from build123d import *

# Parameters (mm, degrees)
SKETCH1_W            = 97.5
SKETCH1_H            = 35
BOSS_EXTRUDE1_DEPTH  = 22
SKETCH2_R            = 3
BOSS_EXTRUDE2_DEPTH  = 4
BOSS_EXTRUDE3_DEPTH  = 2
BOSS_EXTRUDE4_DEPTH  = 8
SKETCH6_R            = 5
BOSS_EXTRUDE5_DEPTH  = 4
SKETCH7_R            = 6.5
SKETCH7_R_2          = 3
BOSS_EXTRUDE6_DEPTH  = 1.5
BOSS_EXTRUDE8_DEPTH  = 8
BOSS_EXTRUDE9_DEPTH  = 4
SKETCH14_R           = 4
BOSS_EXTRUDE10_DEPTH = 2
SKETCH20_R           = 5
BOSS_EXTRUDE11_DEPTH = 4
SKETCH21_R           = 6
SKETCH21_R_2         = 3
BOSS_EXTRUDE12_DEPTH = 1.5
SKETCH22_R           = 2
CUT_EXTRUDE1_DEPTH   = 28.5
SKETCH25_R           = 1.5
CUT_EXTRUDE3_DEPTH   = 39


with BuildPart() as part:
    # Sketch1 → Boss-Extrude1 (new body)
    with BuildSketch(Plane.XY):
        Rectangle(SKETCH1_W, SKETCH1_H)
    extrude(amount=BOSS_EXTRUDE1_DEPTH)

    # Sketch2 → Boss-Extrude2 (add)
    with BuildSketch(Plane(origin=(0, 17.5, 0), x_dir=(1, 0, 0), z_dir=(0, 1, 0))):
        with Locations((-36.875, -11)):
            Circle(SKETCH2_R)
        with Locations((36.875, -11)):
            Circle(SKETCH2_R)
    extrude(amount=BOSS_EXTRUDE2_DEPTH)

    # Sketch3 → Boss-Extrude3 (add)
    with BuildSketch(Plane(origin=(0, 21.5, 0), x_dir=(1, 0, 0), z_dir=(0, 1, 0))):
        with BuildLine():
            Line((37.375, -4), (36.375, -4))
            Line((36.375, -4), (34.078450474, -9.914039252))
            ThreePointArc((34.078450474, -9.914039252), (36.875, -14), (39.671549526, -9.914039252))
            Line((39.671549526, -9.914039252), (37.375, -4))
        make_face()
        with BuildLine():
            Line((-37.364008965, -18.083081838), (-36.368911019, -17.984187559))
            Line((-36.368911019, -17.984187559), (-34.072361493, -12.070148307))
            ThreePointArc((-34.072361493, -12.070148307), (-36.928299188, -8.000473505), (-39.637849875, -12.169042586))
            Line((-39.637849875, -12.169042586), (-37.364008965, -18.083081838))
        make_face()
    extrude(amount=BOSS_EXTRUDE3_DEPTH)

    # Sketch4 → Boss-Extrude4 (add)
    with BuildSketch(Plane(origin=(0, 17.5, 0), x_dir=(1, 0, 0), z_dir=(0, 1, 0))):
        Polygon((-18.080730298, -4.902882533), (-20.354117415, -12.659495476), (-14.773387117, -18.506612943), (-6.919269702, -16.597117467), (-4.645882585, -8.840504524), (-10.226612883, -2.993387057), align=None)
        Polygon((8.255747213, -3.871071914), (4.420547133, -10.98616669), (8.66479992, -17.865094776), (16.744252787, -17.628928086), (20.579452867, -10.51383331), (16.33520008, -3.634905224), align=None)
    extrude(amount=BOSS_EXTRUDE4_DEPTH)

    # Sketch6 → Boss-Extrude5 (add)
    with BuildSketch(Plane(origin=(0, 25.5, 0), x_dir=(1, 0, 0), z_dir=(0, 1, 0))):
        with Locations(Location((-12.5, -10.75, 0), (0, 0, 180))):
            Circle(SKETCH6_R)
        with Locations(Location((12.295473647, -10.75, 0), (0, 0, 180))):
            Circle(SKETCH6_R)
    extrude(amount=BOSS_EXTRUDE5_DEPTH)

    # Sketch7 → Boss-Extrude6 (add)
    # profile 1 of 2: a face of its own
    with BuildSketch(Plane(origin=(0, 29.5, 0), x_dir=(1, 0, 0), z_dir=(0, 1, 0))):
        with Locations(Location((-12.5, -10.75, 0), (0, 0, 180))):
            Circle(SKETCH7_R)
        with Locations(Location((-12.5, -10.75, 0), (0, 0, 180))):
            Circle(SKETCH7_R_2, mode=Mode.SUBTRACT)
    # profile 2 of 2: a face of its own
    with BuildSketch(Plane(origin=(0, 29.5, 0), x_dir=(1, 0, 0), z_dir=(0, 1, 0))):
        with Locations(Location((12.295473647, -10.75, 0), (0, 0, 180))):
            Circle(SKETCH7_R)
        with Locations(Location((12.295473647, -10.75, 0), (0, 0, 180))):
            Circle(SKETCH7_R_2, mode=Mode.SUBTRACT)
    extrude(amount=BOSS_EXTRUDE6_DEPTH)

    # Sketch9 → Boss-Extrude8 (add)
    with BuildSketch(Plane.XZ.offset(17.5)):
        Polygon((-7.809183897, 13.085660615), (-5.710827024, 5.27987867), (2.098356873, 3.194218055), (7.809183897, 8.914339385), (5.710827024, 16.72012133), (-2.098356873, 18.805781945), align=None)
    extrude(amount=BOSS_EXTRUDE8_DEPTH)

    # Sketch13 → Boss-Extrude9 (add)
    with BuildSketch(Plane.XZ.offset(17.5)):
        Polygon((-22.734354602, 6.861918558), (-16.5, 3.839862519), (-10.765645398, 7.727943962), (-11.265645398, 14.638081442), (-17.5, 17.660137481), (-23.234354602, 13.772056038), align=None)
        Polygon((17.5, 17.660137481), (11.265645398, 14.638081442), (10.765645398, 7.727943962), (16.5, 3.839862519), (22.734354602, 6.861918558), (23.234354602, 13.772056038), align=None)
    extrude(amount=BOSS_EXTRUDE9_DEPTH)

    # Sketch14 → Boss-Extrude10 (add)
    with BuildSketch(Plane.XZ.offset(21.5)):
        with Locations((-17, 10.75)):
            Circle(SKETCH14_R)
        with Locations(Location((17, 10.75, 0), (0, 0, 180))):
            Circle(SKETCH14_R)
    extrude(amount=BOSS_EXTRUDE10_DEPTH)

    # Loft1: read off the stored shape, not the designer's step
    # Loft1: loft between two sections, ruled curve by curve
    loft1_from = [
        Edge.make_bspline([(-20.460745722, -23.5, 8.744198652), (-16.449143026, -23.5, 1.822707208), (-9.527651582, -23.5, 5.834309904), (-13.539254278, -23.5, 12.755801348), (-17.550856974, -23.5, 19.677292792), (-24.472348418, -23.5, 15.665690096), (-20.460745722, -23.5, 8.744198652)], [0, 0, 0, 0, 0.5, 0.5, 0.5, 1, 1, 1, 1], 3, [1, 0.333333333, 0.333333333, 1, 0.333333333, 0.333333333, 1]),
    ]
    loft1_to = [
        Edge.make_bspline([(-18.191787926, -33.5, 7.459157928), (-11.610103782, -33.5, 5.075582077), (-9.226527931, -33.5, 11.65726622), (-15.808212074, -33.5, 14.040842072), (-22.389896218, -33.5, 16.424417923), (-24.773472069, -33.5, 9.84273378), (-18.191787926, -33.5, 7.459157928)], [0, 0, 0, 0, 0.5, 0.5, 0.5, 1, 1, 1, 1], 3, [1, 0.333333333, 0.333333333, 1, 0.333333333, 0.333333333, 1]),
    ]
    loft1 = Solid(Shell([*[Face.make_surface_from_curves(loft1_from[k], loft1_to[k]) for k in range(1)], Face(Wire(loft1_from)), Face(Wire(loft1_to))]))
    add(loft1)

    # Loft4: read off the stored shape, not the designer's step
    # Loft4: loft between two sections, ruled curve by curve
    loft4_from = [
        Edge.make_bspline([(16.912042496, -23.5, 6.750967182), (24.910108131, -23.5, 6.575052174), (25.08602314, -23.5, 14.573117809), (17.087957504, -23.5, 14.749032818), (9.089891869, -23.5, 14.924947826), (8.91397686, -23.5, 6.926882191), (16.912042496, -23.5, 6.750967182)], [0, 0, 0, 0, 0.5, 0.5, 0.5, 1, 1, 1, 1], 3, [1, 0.333333333, 0.333333333, 1, 0.333333333, 0.333333333, 1]),
    ]
    loft4_to = [
        Edge.make_bspline([(17.849097308, -33.5, 7.354556912), (24.639983483, -33.5, 9.052751528), (22.941788868, -33.5, 15.843637703), (16.150902692, -33.5, 14.145443088), (9.360016517, -33.5, 12.447248472), (11.058211132, -33.5, 5.656362297), (17.849097308, -33.5, 7.354556912)], [0, 0, 0, 0, 0.5, 0.5, 0.5, 1, 1, 1, 1], 3, [1, 0.333333333, 0.333333333, 1, 0.333333333, 0.333333333, 1]),
    ]
    loft4 = Solid(Shell([*[Face.make_surface_from_curves(loft4_from[k], loft4_to[k]) for k in range(1)], Face(Wire(loft4_from)), Face(Wire(loft4_to))]))
    add(loft4)

    # Sketch20 → Boss-Extrude11 (add)
    with BuildSketch(Plane.XZ.offset(25.5)):
        with Locations((0, 11)):
            Circle(SKETCH20_R)
    extrude(amount=BOSS_EXTRUDE11_DEPTH)

    # Sketch21 → Boss-Extrude12 (add)
    with BuildSketch(Plane(origin=(0, -29.5, 0), x_dir=(-1, 0, 0), z_dir=(0, -1, 0))):
        with Locations(Location((0, -11, 0), (0, 0, 180))):
            Circle(SKETCH21_R)
        with Locations(Location((0, -11, 0), (0, 0, 180))):
            Circle(SKETCH21_R_2, mode=Mode.SUBTRACT)
    extrude(amount=BOSS_EXTRUDE12_DEPTH)

    # Sketch22 → Cut-Extrude1 (cut)
    with BuildSketch(Plane.XY.offset(22)):
        with Locations((-9.75, -8.5)):
            Circle(SKETCH22_R)
        with Locations((9.75, -8.5)):
            Circle(SKETCH22_R)
    extrude(amount=-CUT_EXTRUDE1_DEPTH, mode=Mode.SUBTRACT)

    # Sketch25 → Cut-Extrude3 (cut)
    with BuildSketch(Plane(origin=(0, 17.5, 0), x_dir=(1, 0, 0), z_dir=(0, 1, 0))):
        with Locations(Location((-21.5, -20, 0), (0, 0, 180))):
            Circle(SKETCH25_R)
        with Locations(Location((21.5, -2, 0), (0, 0, 180))):
            Circle(SKETCH25_R)
    extrude(amount=-CUT_EXTRUDE3_DEPTH, mode=Mode.SUBTRACT)


solid = part.part
CAD build for the part. Positions are in the model's coordinates, mm. A direction names the side the tool comes from. Round coordinates to 2 decimals unless told otherwise and drop trailing zeros. Write each loop counter-clockwise with the first axis right and the second up, starting at its lowest first coordinate (ties: lowest second). Pieces come first, ordered by that corner, then holes. Notation, with made-up numbers: M -2.5,-38.5 L 24.5,-38.5 A10 ccw 24.5,-21.5 Z; hole C 9,19 d2. An arc over 180 degrees is marked long. Use a Markdown table: item, result. Add a question column.
1. Slice it at A-A on y = -8.5. Give the cut face in (x, z), then the cut area to 3 significant figures.
2. Drill centre lines: probe 1 along X at (y, z) = (-23, 9.75); probe 2 along X at (y, z) = (-7, 4.5); probe 3 along Y at (x, z) = (9.75, 8.5). Where is each one in solid material? Low to high.
3. Slice it at C-C on x = -1. Give the cut face in (y, z), then the cut area to 3 significant figures.
4. Flat gauge pins, fed straight in: P1, Ø0.5, axis at x = 37, y = 22.5, coming from the -Z side; P2, Ø2.5, axis at x = -21.5, z = 20, coming from the -Y side; P3, Ø1.7, axis at x = -37.5, z = 14.5, coming from the -Y side; P4, Ø6.5, axis at x = 1, z = 10, coming from the -Y side. Where does each tip first touch, or does it go through?
5. 3-axis set-ups, long thin cutter, end or side, ignore diameter. For faces 3 (the face through (8, 29.5, 7)), 4 (the face through (-17.603, 21.444, 15.542)), 5 (the face through (1, -31, 14)), 6 (the face through (6.096, 30.24, 12.702)), 7 (the face through (-1.301, -30.24, 5.143)): which of +Z, -Z, +X, -X, +Y, -Y reach the whole face in a straight line?
6. Slice it at B-B on z = 20. Give the cut face in (x, y), then the cut area to 3 significant figures.
7. Pull direction X, two halves, no side cores. Call faces 1 (the face through (-4, -29.5, 15)), 2 (the face through (-14.099, 21.444, 3.935)): released by +X, released by -X, zero draft, split by the parting line, or undercut.
Reply:
| question | item | result |
|---|---|---|
| 1 | outline | M -48.75,0 L -11.75,0 L -11.75,22 L -48.75,22 Z; M -7.75,0 L 7.75,0 L 7.75,22 L -7.75,22 Z; M 11.75,0 L 48.75,0 L 48.75,22 L 11.75,22 Z; hole C -21.5,20 d3; hole C 21.5,2 d3 |
| 1 | area | 1,950 mm^2 |
| 2 | probe 1 | x = -20.87 to -13.13, -6.91 to 7.58, 13.13 to 20.87 |
| 2 | probe 2 | x = -48.75 to -11.07, -8.43 to 8.43, 11.07 to 48.75 |
| 2 | probe 3 | y = -17.5 to -10.5, -6.5 to 31 |
| 3 | outline | M -31,5.08 L -29.5,5.08 L -29.5,6.1 L -25.5,6.1 L -25.5,4.02 L -17.5,4.02 L -17.5,0 L 17.5,0 L 17.5,22 L -17.5,22 L -17.5,18.51 L -25.5,18.51 L -25.5,15.9 L -29.5,15.9 L -29.5,16.92 L -31,16.92 L -31,13.83 L -29.5,13.83 L -29.5,8.17 L -31,8.17 Z |
| 3 | area | 934 mm^2 |
| 4 | P1 | stops at z = 4 |
| 4 | P2 | passes through |
| 4 | P3 | stops at y = -17.5 |
| 4 | P4 | stops at y = -31 |
| 5 | face 3 | none |
| 5 | face 4 | +Z, +Y |
| 5 | face 5 | +Z, -Z, -Y |
| 5 | face 6 | +Y |
| 5 | face 7 | -Y |
| 6 | outline | M -48.75,-17.5 L -23,-17.5 L -23,17.5 L -48.75,17.5 Z; M -20,-17.5 L 48.75,-17.5 L 48.75,17.5 L -20,17.5 Z; hole C -9.75,-8.5 d4; hole C 9.75,-8.5 d4 |
| 6 | area | 3,280 mm^2 |
| 7 | face 1 | undercut |
| 7 | face 2 | released by -X |
